Check sheet for the modelled part. Datum: model origin and axes. Units: mm. Coordinates: 2 decimals unless noted, no trailing zeros. Loops run counter-clockwise (first coordinate to the right, second up) from the corner with the lowest first, then second, coordinate; pieces in that order, holes last. Notation, with made-up numbers: M 16.25,-23.75 L 57.25,-23.75 A29 ccw 57.25,-1.75 Z; hole C -37.5,-8.5 d5. An arc over 180 degrees is marked long. Return JSON: item names as keys, results as strings.
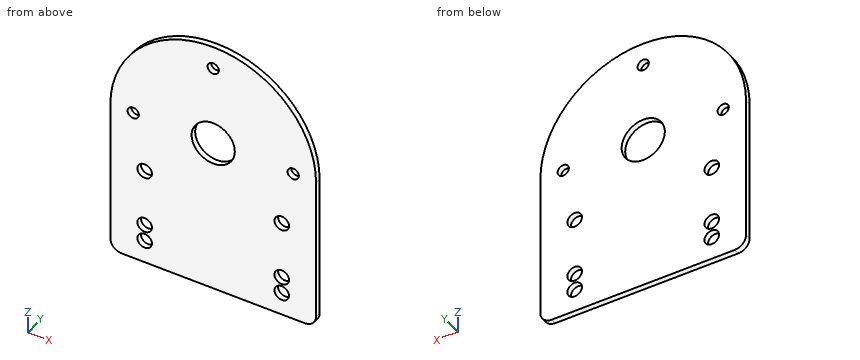
from build123d import *

# Parameters (mm, degrees)
SKETCH1_R           = 6
SKETCH1_R_2         = 1.5625
SKETCH1_R_3         = 2.025
BOSS_EXTRUDE1_DEPTH = 1.5875


with BuildPart() as part:
    # Sketch1 → Boss-Extrude1 (new body)
    with BuildSketch(Plane(origin=(0, 0, 0), x_dir=(1, 0, 0), z_dir=(0, 1, 0))):
        with BuildLine():
            Line((-28.575, 0), (-28.575, 39.875))
            ThreePointArc((-28.575, 39.875), (-27.64506403, 42.12006403), (-25.4, 43.05))
            Line((-25.4, 43.05), (25.4, 43.05))
            ThreePointArc((25.4, 43.05), (27.64506403, 42.12006403), (28.575, 39.875))
            Line((28.575, 39.875), (28.575, 0))
            ThreePointArc((28.575, 0), (0, -28.575), (-28.575, 0))
        make_face()
        Circle(SKETCH1_R, mode=Mode.SUBTRACT)
        with Locations((-22.225, 0)):
            Circle(SKETCH1_R_2, mode=Mode.SUBTRACT)
        with Locations((0, -22.225)):
            Circle(SKETCH1_R_2, mode=Mode.SUBTRACT)
        with Locations((22.225, 0)):
            Circle(SKETCH1_R_2, mode=Mode.SUBTRACT)
        with Locations((-19.05, 16)):
            Circle(SKETCH1_R_3, mode=Mode.SUBTRACT)
        with Locations((19.05, 16)):
            Circle(SKETCH1_R_3, mode=Mode.SUBTRACT)
        with Locations((19.05, 32)):
            Circle(SKETCH1_R_3, mode=Mode.SUBTRACT)
        with Locations((-19.05, 32)):
            Circle(SKETCH1_R_3, mode=Mode.SUBTRACT)
        with Locations((-19.05, 36.7)):
            Circle(SKETCH1_R_3, mode=Mode.SUBTRACT)
        with Locations((19.05, 36.7)):
            Circle(SKETCH1_R_3, mode=Mode.SUBTRACT)
    extrude(amount=BOSS_EXTRUDE1_DEPTH)


solid = part.part
1) Section check B-B on x = 0. Count the separate pieces of the cut face and the enclosed holes in it, then the cut area to 3 significant figures.
Answers:
{"separate pieces": "3", "enclosed holes": "0", "area": "89.7 mm²"}
2) Section check D-D on x = -18. Record the cut outline in (y, z).
Answers:
{"outline": "M 0,-43.05 L 1.59,-43.05 L 1.59,-38.43 L 0,-38.43 Z; M 0,-34.97 L 1.59,-34.97 L 1.59,-33.73 L 0,-33.73 Z; M 0,-30.27 L 1.59,-30.27 L 1.59,-17.73 L 0,-17.73 Z; M 0,-14.27 L 1.59,-14.27 L 1.59,22.19 L 0,22.19 Z"}
3) Section check A-A on z = -32. Record the cut outline in (x, y) (1 decimal), then the cut area to 3 significant figures.
Answers:
{"outline": "M -28.6,0 L -21.1,0 L -21.1,1.6 L -28.6,1.6 Z; M -17,0 L 17,0 L 17,1.6 L -17,1.6 Z; M 21.1,0 L 28.6,0 L 28.6,1.6 L 21.1,1.6 Z", "area": "77.9 mm²"}
4) Scan lines: line 1 along X through (y, z) = (1.15, -36.7) (3 decimals); line 2 along Z through (x, y) = (20.5, 0.75); line 3 along X through (y, z) = (1.4, -38) (3 decimals). Record each from-to range of solid material in increasing order. Write a range as [from, to].
Answers:
{"line 1": "[-28.575, -21.075], [-17.025, 17.025], [21.075, 28.575]", "line 2": "[-43.05, -38.11], [-35.29, -33.41], [-30.59, -17.41], [-14.59, 19.91]", "line 3": "[-28.575, -20.603], [-17.497, 17.497], [20.603, 28.575]"}
5) Go/stop test with flat-tipped pins: pin 1 Ø10 at (x, z) = (-16.5, -15.5) entering from -Y; pin 2 Ø3 at (x, z) = (-19.05, -32) entering from -Y. Record where each tip stops, or that it passes through.
Answers:
{"pin 1": "y = 0", "pin 2": "through"}
